Geometry check sheet. Reference: the model listing, model coordinates, mm. A direction names the side the tool comes from. Coordinates: 2 decimals unless noted, no trailing zeros. Write each loop counter-clockwise with the first axis right and the second up, starting at its lowest first coordinate (ties: lowest second). Pieces come first, ordered by that corner, then holes. Notation, with made-up numbers: M -10,31 L 6,31 A12 ccw 6,46 Z; hole C -35.75,72.5 d10. An arc over 180 degrees is marked long. Write item = value, one per line. Start each with the question number.
```python
from build123d import *

# Parameters (mm, degrees)
ESQUISSE1_R        = 5
ESQUISSE1_R_2      = 1.5
ESQUISSE1_R_3      = 2
BOSS_EXTRU_1_DEPTH = 2


with BuildPart() as part:
    # Esquisse1 → Boss.-Extru.1 (new body)
    with BuildSketch(Plane.XY):
        with BuildLine():
            Line((18, -6.5), (18, -13))
            ThreePointArc((18, -13), (21.5, -16.5), (25, -13))
            Line((25, -13), (25, -6.5))
            ThreePointArc((25, -6.5), (26.464466094, -2.964466094), (30, -1.5))
            Line((30, -1.5), (36.5, -1.5))
            ThreePointArc((36.5, -1.5), (40, 2), (36.5, 5.5))
            Line((36.5, 5.5), (30, 5.5))
            ThreePointArc((30, 5.5), (26.464466094, 6.964466094), (25, 10.5))
            Line((25, 10.5), (25, 17))
            ThreePointArc((25, 17), (21.5, 20.5), (18, 17))
            Line((18, 17), (18, 10.5))
            ThreePointArc((18, 10.5), (16.535533906, 6.964466094), (13, 5.5))
            Line((13, 5.5), (6.5, 5.5))
            ThreePointArc((6.5, 5.5), (3, 2), (6.5, -1.5))
            Line((6.5, -1.5), (13, -1.5))
            ThreePointArc((13, -1.5), (16.535533906, -2.964466094), (18, -6.5))
        make_face()
        with Locations((21.5, 2)):
            Circle(ESQUISSE1_R, mode=Mode.SUBTRACT)
        with Locations((12.5, 2)):
            Circle(ESQUISSE1_R_2, mode=Mode.SUBTRACT)
        with Locations((6.5, 2)):
            Circle(ESQUISSE1_R_3, mode=Mode.SUBTRACT)
        with Locations((21.5, 17)):
            Circle(ESQUISSE1_R_3, mode=Mode.SUBTRACT)
        with Locations((21.5, 11)):
            Circle(ESQUISSE1_R_2, mode=Mode.SUBTRACT)
        with Locations((36.5, 2)):
            Circle(ESQUISSE1_R_3, mode=Mode.SUBTRACT)
        with Locations((30.5, 2)):
            Circle(ESQUISSE1_R_2, mode=Mode.SUBTRACT)
        with Locations((21.5, -13)):
            Circle(ESQUISSE1_R_3, mode=Mode.SUBTRACT)
        with Locations((21.5, -7)):
            Circle(ESQUISSE1_R_2, mode=Mode.SUBTRACT)
    extrude(amount=BOSS_EXTRU_1_DEPTH)


solid = part.part
```
Q1. Draft check along Y on faces 1 (the face through (10, 5.5, 1)), 2 (the face through (20, 11, 1)), 3 (the face through (10, -1.5, 1)). Enter one of: pulls with the +Y half, pulls with the -Y half, needs draft (parallel to the pull), parting line crosses it, or undercut.
Q2. Scan lines: L1, parallel to Y at x = 21.5, z = 0.8; L2, parallel to Y at x = 36.5, z = 0.5; L3, parallel to Y at x = 17.5, z = 1.5. Record each from-to range of solid material in increasing order.
Q3. Cross-section at D-D on z = 0.7. Count the separate pieces of the cut face and the enclosed holes in it, and give its area (3 significant figures).
Q4. Set-up check for faces 4 (the face through (25, -10, 1)), 5 (the face through (18, 14, 1)), 6 (the face through (25, 14, 1)): record each of +Z, -Z, +X, -X, +Y, -Y from which the full face is reachable in a straight line by a thin tool's end or side.
Q5. Cross-section at A-A on x = 21.5. Enter the section's corners in (y, z).
Q6. Cross-section at B-B on y = 2. Enter the section's corners in (x, z).
Q7. Gauge pin test, flat ends, axial feed: pin 1 (1 mm diameter, centred on y = 12, z = 1, fed in from +X); pin 2 (1 mm diameter, centred on x = 10.5, z = 0.5, fed in from +Y); pin 3 (1 mm diameter, centred on y = -4.5, z = 1.5, fed in from -X). Record the tip position at first contact, or that the pin passes through.
Q8. Cross-section at C-C on x = 30.5. Enter the section's corners in (y, z), and give its area (3 significant figures).
Values found:
q1.face_1 = pulls with the +Y half
q1.face_2 = undercut
q1.face_3 = pulls with the -Y half
q2.L1 = -16.5 to -15, -11 to -8.5, -5.5 to -3, 7 to 9.5, 12.5 to 15, 19 to 20.5
q2.L2 = -1.5 to 0, 4 to 5.5
q2.L3 = -4.32 to -1, 5 to 8.32
q3.separate_pieces = 1
q3.enclosed_holes = 9
q3.area = 312 mm²
q4.face_4 = +Z, -Z, +X, -Y
q4.face_5 = +Z, -Z, -X, +Y
q4.face_6 = +Z, -Z, +X, +Y
q5.outline = M -16.5,0 L -15,0 L -15,2 L -16.5,2 Z; M -11,0 L -8.5,0 L -8.5,2 L -11,2 Z; M -5.5,0 L -3,0 L -3,2 L -5.5,2 Z; M 7,0 L 9.5,0 L 9.5,2 L 7,2 Z; M 12.5,0 L 15,0 L 15,2 L 12.5,2 Z; M 19,0 L 20.5,0 L 20.5,2 L 19,2 Z
q6.outline = M 3,0 L 4.5,0 L 4.5,2 L 3,2 Z; M 8.5,0 L 11,0 L 11,2 L 8.5,2 Z; M 14,0 L 16.5,0 L 16.5,2 L 14,2 Z; M 26.5,0 L 29,0 L 29,2 L 26.5,2 Z; M 32,0 L 34.5,0 L 34.5,2 L 32,2 Z; M 38.5,0 L 40,0 L 40,2 L 38.5,2 Z
q7.pin_1 = 25
q7.pin_2 = 5.5
q7.pin_3 = 17.33
q8.outline = M -1.5,0 L 0.5,0 L 0.5,2 L -1.5,2 Z; M 3.5,0 L 5.5,0 L 5.5,2 L 3.5,2 Z
q8.area = 8.00 mm²
